Design review of the part built by this model. Coordinates are the model's own, in mm. Face numbers are marked on the shaded views. A direction names the side the tool comes from. Coordinates: 2 decimals unless noted, no trailing zeros. Loops run counter-clockwise (first coordinate to the right, second up) from the corner with the lowest first, then second, coordinate; pieces in that order, holes last. Notation, with made-up numbers: M 63,-1.5 L 113,-1.5 A13 cw 113,19.5 Z; hole C 77,45 d11. An arc over 180 degrees is marked long. One line per item, written item: value.
```python
from build123d import *

# Parameters (mm, degrees)
BOSS_EXTRUDE1_DEPTH      = 7
BOSS_EXTRUDE2_DEPTH      = 1
BOSS_EXTRUDE3_DEPTH      = 2.5
BOSS_EXTRUDE3_DEPTH_BACK = 2.5
CUT_EXTRUDE1_DEPTH       = 7


with BuildPart() as part:
    # Sketch1 → Boss-Extrude1 (new body)
    with BuildSketch(Plane(origin=(0, 0, 0), x_dir=(1, 0, 0), z_dir=(0, 1, 0))):
        with BuildLine():
            Line((-1, -4.387482194), (-1, -3.354101966))
            ThreePointArc((-1, -3.354101966), (-2.091650066, 2.80624304), (3.5, 0))
            ThreePointArc((3.5, 0), (2.80624304, -2.091650066), (1, -3.354101966))
            Line((1, -3.354101966), (1, -4.387482194))
            ThreePointArc((1, -4.387482194), (3.51781182, -2.80624304), (4.5, 0))
            ThreePointArc((4.5, 0), (-2.80624304, 3.51781182), (-1, -4.387482194))
        make_face()
    extrude(amount=BOSS_EXTRUDE1_DEPTH)

    # Sketch2 → Boss-Extrude2 (add)
    with BuildSketch(Plane(origin=(0, 7, 0), x_dir=(1, 0, 0), z_dir=(0, 1, 0))):
        with BuildLine():
            Line((-1, -3.354101966), (-1, 0))
            ThreePointArc((-1, 0), (0, 1), (1, 0))
            Line((1, 0), (1, -3.354101966))
            ThreePointArc((1, -3.354101966), (0, 3.5), (-1, -3.354101966))
        make_face()
        with BuildLine():
            ThreePointArc((-1, -3.354101966), (0, 3.5), (1, -3.354101966))
            Line((1, -3.354101966), (1, -4.387482194))
            ThreePointArc((1, -4.387482194), (0, 4.5), (-1, -4.387482194))
            Line((-1, -4.387482194), (-1, -3.354101966))
        make_face()
    extrude(amount=BOSS_EXTRUDE2_DEPTH)

    # Sketch3 → Boss-Extrude3 (add, two sides: drawn at the far end of the back side and taken through both)
    with BuildSketch(Plane(origin=(0, 0, 0), x_dir=(0, 0, -1), z_dir=(1, 0, 0)).offset(-BOSS_EXTRUDE3_DEPTH_BACK)):
        Polygon((7.5, 6), (4.5, 6), (3.5, 6), (3.5, 2), (7.5, 2), align=None)
    extrude(amount=BOSS_EXTRUDE3_DEPTH + BOSS_EXTRUDE3_DEPTH_BACK)

    # Sketch4 → Cut-Extrude1 (cut)
    with BuildSketch(Plane(origin=(0, 6, 0), x_dir=(1, 0, 0), z_dir=(0, 1, 0))):
        Polygon((1.75, 6.8), (0, 6.8), (-1.75, 6.8), (-1.75, 5.7), (1.75, 5.7), align=None)
    extrude(amount=-CUT_EXTRUDE1_DEPTH, mode=Mode.SUBTRACT)


solid = part.part
```
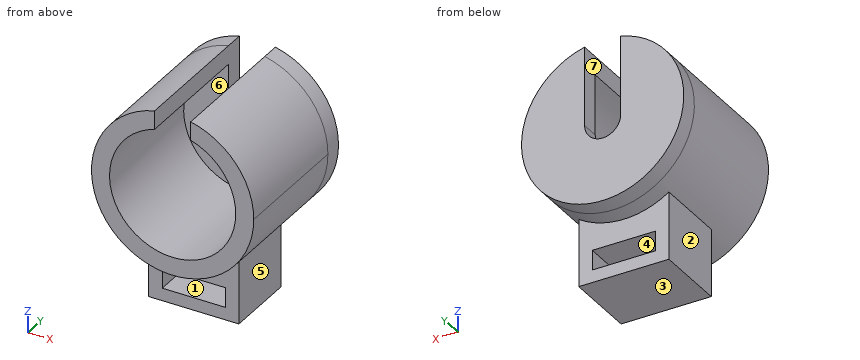
(1) To check wall thickness, follow line 1 along X through (y, z) = (3.25, 0); line 2 along Y through (x, z) = (1.25, 2.5); line 3 along X through (y, z) = (2.25, -4.75). State the ranges of each line that lie inside material, in increasing order. Write a range as [from, to].
Reply:
line 1: x = [-4.5, -3.5], [3.5, 4.5]
line 2: y = [7, 8]
line 3: x = [-2.5, 2.5]
(2) Mouldability with a two-part tool opening along X and no side actions: class the marked faces 1, 2 and 3 as released by +X, released by -X, zero draft, split by the parting line, or undercut.
Reply:
face 1: undercut
face 2: released by -X
face 3: zero draft
(3) We need section A-A on x = 0. State the section outline as (y, z) points, then the cut area to 3 significant figures.
Reply:
outline: M 0,-4.5 L 2,-4.5 L 2,-5.7 L 6,-5.7 L 6,-4.5 L 8,-4.5 L 8,-1 L 7,-1 L 7,-3.5 L 0,-3.5 Z; M 2,-7.5 L 6,-7.5 L 6,-6.8 L 2,-6.8 Z
area: 18.1 mm2
(4) Insertion check: pin 1 (3 mm diameter, centred on y = 4.5, z = -6, fed in from -X); pin 2 (1.9 mm diameter, centred on x = -1, z = -6, fed in from +Y); pin 3 (1.5 mm diameter, centred on y = 5.5, z = 3, fed in from -X). Each pin has a flat end and moves straight along its axis. Give the tip position at first contact, or say it passes through.
Reply:
pin 1: stops at x = -2.5
pin 2: stops at y = 6
pin 3: stops at x = -3.9
(5) We need section B-B on y = 3. State the section outline as (x, z) points.
Reply:
outline: M -2.5,-7.5 L 2.5,-7.5 L 2.5,-3.74 A4.5 ccw 1,4.39 L 1,3.35 A3.5 cw long -1,3.35 L -1,4.39 A4.5 ccw -2.5,-3.74 Z; hole M -1.75,-6.8 L 1.75,-6.8 L 1.75,-5.7 L -1.75,-5.7 Z
(6) Tool access review of the marked faces 4, 5, 6 and 7: name each direction out of +Z, -Z, +X, -X, +Y, -Y from which nothing blocks a thin tool from reaching the whole face with its end or side.
Reply:
face 4: +Y, -Y
face 5: -Z, +X, +Y, -Y
face 6: -Y
face 7: +Z, +Y, -Y
(7) We need section D-D on x = 3.25. State the section outline as (y, z) points, then the cut area to 3 significant figures.
Reply:
outline: M 0,-3.11 L 8,-3.11 L 8,3.11 L 0,3.11 L 0,1.3 L 7,1.3 L 7,-1.3 L 0,-1.3 Z
area: 31.6 mm2
(8) We need section C-C on z = 1.5. State the section outline as (x, y) points.
Reply:
outline: M -4.24,0 L -3.16,0 L -3.16,7 L -1,7 L -1,8 L -4.24,8 Z; M 1,7 L 3.16,7 L 3.16,0 L 4.24,0 L 4.24,8 L 1,8 Z
